Read the model definition and answer for the solid it produces. Units are mm, in the model's axes. Give positions to 0.01 mm unless a question says otherwise; leave off trailing zeros. Write each loop counter-clockwise with the first axis right and the second up, starting at its lowest first coordinate (ties: lowest second). Pieces come first, ordered by that corner, then holes. Notation, with made-up numbers: M -29,56 L -17,56 A35 cw -17,95 Z; hole C 44,-26 d10. An arc over 180 degrees is marked long. Put each result on its own line as item: value.
Autodesk Inventor part; units mm, degrees
ref_plane "YZ Plane" through (0, 0, 0) normal (1, 0, 0) x (0, 1, 0)
ref_plane "XZ Plane" through (0, 0, 0) normal (0, 1, 0) x (-1, 0, 0)
ref_plane "XY Plane" through (0, 0, 0) normal (0, 0, 1) x (1, 0, 0)
sketch "Sketch the Prototype Plate Base Profile" plane through (0, 0, 0) normal (0, 0, 1) x (1, 0, 0)
  circle A0 centre (0, 0) radius 137
  dimension "d0" = 274
extrude "Make Prototype Plate Base by Extrusion" add sketch "Sketch the Prototype Plate Base Profile" along normal mid plane 9
sketch "Locate the Outer Rib Slots" plane through (0, 0, 4.5) normal (0, 0, 1) x (1, 0, 0)
  circle A0 centre (0, 0) radius 137
  line L0 (0, 0) -> (0, 137) construction
  circle A1 centre (0, 137) radius 15 construction
  line L1 (-24, 118.2578) -> (-15, 118.2578)
  line L2 (-15, 118.2578) -> (-15, 98.2578)
  line L3 (-15, 98.2578) -> (-24, 98.2578)
  line L4 (-24, 98.2578) -> (-24, 118.2578)
  line L5 (-24, 118.2578) -> (-15, 98.2578) construction
  line L6 (-15, 118.2578) -> (-24, 98.2578) construction
  line L7 (-19.5, 108.2578) -> (-15, 108.2578) construction
  circle A2 centre (0, 0) radius 61 construction
  line L8 (24, 118.2578) -> (15, 118.2578)
  line L9 (15, 118.2578) -> (15, 98.2578)
  line L10 (15, 98.2578) -> (24, 98.2578)
  line L11 (24, 98.2578) -> (24, 118.2578)
  circle A3 centre (0, 0) radius 110 construction
  line L12 (-15, 98.2578) -> (0, 98.2578) construction
  dimension "d29" = 220
  dimension "d3" = 30
  dimension "d5" = 20
  dimension "d15" = 9
  dimension "d17" = 122
  dimension "d30" = 15
extrude "Cut Outer Rib Slots" cut sketch "Locate the Outer Rib Slots" against normal blind 9 contours L1 L2 L3 L4 | L11 L10 L9 L8
pattern_circular "Pattern Outer Rib Slots Around the Base Plate" count 3 over 360 about axis through (0, 0, -10) along (0, 0, 1) of "Cut Outer Rib Slots"
sketch "Locate the Inner Rib Slot" plane through (0, 0, 4.5) normal (0, 0, 1) x (1, 0, 0)
  circle A0 centre (0, 0) radius 137
  line L0 (-106.173, 56.1029) -> (-101.673, 63.8971)
  line L1 (-101.673, 63.8971) -> (-84.3525, 53.8971)
  line L2 (-84.3525, 53.8971) -> (-88.8525, 46.1029)
  line L3 (-88.8525, 46.1029) -> (-106.173, 56.1029)
  line L4 (-106.173, 56.1029) -> (-84.3525, 53.8971) construction
  line L5 (-101.673, 63.8971) -> (-88.8525, 46.1029) construction
  circle A1 centre (0, 0) radius 110 construction
  line L6 (-95.2628, 55) -> (0, 0) construction
  line L7 (0, -210.7) -> (0, 210.7)
  dimension "d31" = 220
  dimension "d27" = 9
  dimension "d28" = 20
  dimension "d32" = 60
extrude "Cut Inner Rib Slots" cut sketch "Locate the Inner Rib Slot" against normal blind 9 contours L0 L1 L2 L3
pattern_circular "Pattern Inner Rib Slots Around the Base Plate" count 3 over 360 about axis through (0, 0, -10) along (0, 0, 1) of "Cut Inner Rib Slots"
sketch "Locate Holes for Connecting Two Bases" plane through (0, 0, 4.5) normal (0, 0, 1) x (1, 0, 0)
  circle A0 centre (0, 0) radius 137
  line L0 (-15, 118.2578) -> (-15, 98.2578)
  line L1 (15, 98.2578) -> (15, 118.2578)
  circle A1 centre (0, 0) radius 110 construction
  line L2 (0, 0) -> (0, 110) construction
  line L3 (-24, 98.2578) -> (-24, 118.2578)
  line L4 (-101.673, 63.8971) -> (-84.3525, 53.8971)
  circle A2 centre (-92.933, 58.8511) radius 42.9699 construction
  circle A3 centre (-24, 107.3499) radius 42.9699 construction
  line L5 (24, 118.2578) -> (24, 98.2578)
  line L6 (84.3525, 53.8971) -> (101.673, 63.8971)
  circle A4 centre (24, 107.3499) radius 42.9699 construction
  circle A5 centre (92.933, 58.8511) radius 42.9699 construction
  point P0 (-63.2959, 89.9646)
  point P1 (63.2959, 89.9646)
  point P2 (-46.2637, -99.7981)
  point P3 (-109.5596, 9.8335)
  point P4 (109.5596, 9.8335)
  point P5 (46.2637, -99.7981)
  dimension "d54" = 220
  dimension "d66" = 360
hole "Clearance Holes to Bolt the Two Bases Together" at (-63.2959, 89.9646, 4.5) at (63.2959, 89.9646, 4.5) at (-46.2637, -99.7981, 4.5) at (-109.5596, 9.8335, 4.5) at (109.5596, 9.8335, 4.5) at (46.2637, -99.7981, 4.5) direction (0, 0, -1) diameter 6.4 end through all
hole "Clearance Holes to Bolt the Two Bases Together at Arms" at (0, 110, 4.5) at (-95.2628, -55, 4.5) at (95.2628, -55, 4.5) direction (0, 0, -1) diameter 6.4 end through all
equation "\"d0\" = PrototypePlateDiameter"
equation "\"d1\" = PrototypePlateMaterialThickness"
equation "\"d29\" = OuterRibSlotPCD"
equation "\"d3\" = RigColumnsDiameter"
equation "\"d5\" = RibSlotLength"
equation "\"d15\" = PrototypePlateRibMaterialThickness"
equation "\"d30\" = 0.5 * RigColumnsDiameter"
equation "\"d18\" = PrototypePlateMaterialThickness"
equation "\"d31\" = InnerRibSlotPCD"
equation "\"d27\" = PrototypePlateRibMaterialThickness"
equation "\"d28\" = RibSlotLength"
equation "\"d33\" = PrototypePlateMaterialThickness"
equation "\"d54\" = InnerRibSlotPCD"
equation "\"d75\" = InnerRibSlotPCD"
properties part number "Prototype Plate Base"
(1) Straight lines are drawn through the part: line 1 along X through (y, z) = (110, -1.75); line 2 along Y through (x, z) = (-104, -1.25); line 3 along X through (y, z) = (90, 3.25). For each, find the intervals that lie inside material, in ascending order. Write a range as from..to.
Result:
line 1: x = -81.66..-24, -15..-3.2, 3.2..15, 24..81.66
line 2: y = -89.18..-42.72, -32.33..54.85, 59.87..89.18
line 3: x = -103.29..-66.5, -60.1..60.1, 66.5..103.29
(2) For a pull along X with two mould halves and no side action, classify faces 1 (the face through (20, 118.258, 0)), 2 (the face through (-2, 2, 4.5)), 3 (the face through (130.674, 41.151, 0.063)) as +X half, -X half, draft (parallel to the pull), parting line (faces both ways), or undercut.
Result:
face 1: undercut
face 2: draft
face 3: parting line
(3) Section B-B on y = 110 is taken. Determine the outline of the cut face in (x, z).
Result:
outline: M -81.66,-4.5 L -24,-4.5 L -24,4.5 L -81.66,4.5 Z; M -15,-4.5 L -3.2,-4.5 L -3.2,4.5 L -15,4.5 Z; M 3.2,-4.5 L 15,-4.5 L 15,4.5 L 3.2,4.5 Z; M 24,-4.5 L 81.66,-4.5 L 81.66,4.5 L 24,4.5 Z
(4) Section A-A on x = 0 is taken. Determine the outline of the cut face in (y, z), and give its area (3 significant figures).
Result:
outline: M -137,-4.5 L -120,-4.5 L -120,4.5 L -137,4.5 Z; M -100,-4.5 L 106.8,-4.5 L 106.8,4.5 L -100,4.5 Z; M 113.2,-4.5 L 137,-4.5 L 137,4.5 L 113.2,4.5 Z
area: 2,230 mm²
(5) Given pin 1 Ø4 at (x, y) = (-95.26, -55) entering from -Z; pin 2 Ø2 at (y, z) = (101, 3.5) entering from +X; pin 3 Ø4.5 at (y, z) = (110, 0) entering from -X; pin 4 Ø4.5 at (x, z) = (17.5, 1.5) entering from +Y, each flat-ended and moving along its own axis, determine where each tip first touches the part or whether it passes through.
Result:
pin 1: passes through
pin 2: stops at x = 93.64
pin 3: stops at x = -84.61
pin 4: stops at y = 136.15
(6) Section D-D on z = 0.75 is taken. Give the number of separate pieces and of enclosed holes in the cut face, and give its area (3 significant figures).
Result:
separate pieces: 1
enclosed holes: 18
area: 57,100 mm²
(7) Section C-C on y = -55 is taken. Determine the outline of the cut face in (x, z), and give its area (3 significant figures).
Result:
outline: M -125.48,-4.5 L -98.46,-4.5 L -98.46,4.5 L -125.48,4.5 Z; M -92.06,-4.5 L 92.06,-4.5 L 92.06,4.5 L -92.06,4.5 Z; M 98.46,-4.5 L 125.48,-4.5 L 125.48,4.5 L 98.46,4.5 Z
area: 2,140 mm²
